Autodesk Inventor part; units mm, degrees
ref_plane "YZ Plane" through (0, 0, 0) normal (1, 0, 0) x (0, 1, 0)
ref_plane "XZ Plane" through (0, 0, 0) normal (0, 1, 0) x (-1, 0, 0)
ref_plane "XY Plane" through (0, 0, 0) normal (0, 0, 1) x (1, 0, 0)
sketch "Sketch1" plane through (0, 0, 0) normal (1, 0, 0) x (0, 1, 0)
  line L0 (-19.6181, -6.8872) -> (-0.5681, -6.8872)
  line L1 (-0.5681, -6.8872) -> (-0.5681, -10.0622)
  line L2 (-0.5681, -10.0622) -> (-19.6181, -10.0622)
  line L3 (-19.6181, -10.0622) -> (-19.6181, -6.8872)
  dimension "d7" = 19.05
  dimension "d8" = 3.175
extrude "Extrusion1" add sketch "Sketch1" along normal blind 38.1
sketch "Sketch2" plane through (0, -0.5681, -6.8872) normal (0, 1, 0) x (1, 0, 0)
  line L0 (38.1, 3.175) -> (38.1, 0)
  arc A0 (38.1, 1.5875) -> (241.3, 1.5875) centre (139.7, 115.1798) ccw
  line L1 (0, 0) -> (38.1, 0)
  point P0 (0, -6.8872)
  dimension "d11" = 203.2
  dimension "d12" = 152.4
  dimension "d17" = 1.5875
sketch "Sketch3" plane through (38.1, 0, 0) normal (1, 0, 0) x (0, 0, -1)
  line L0 (6.8872, -0.5681) -> (6.8872, -19.6181)
  line L1 (6.8872, -19.6181) -> (10.0622, -19.6181)
  line L2 (10.0622, -19.6181) -> (10.0622, -0.5681)
  line L3 (10.0622, -0.5681) -> (6.8872, -0.5681)
  point P0 (0, 0)
sweep "Sweep1" add profiles "Sketch3" path "Sketch2" path curves A0
sketch "Sketch4" plane through (0, -0.5681, -6.8872) normal (0, 1, 0) x (1, 0, 0)
  line L0 (239.7223, 1.7639) -> (242.8777, 1.4111)
  line L1 (0, 3.175) -> (38.1, 3.175)
  line L2 (239.7223, 1.7639) -> (239.7223, 20.8139)
  line L3 (239.7223, 20.8139) -> (242.8777, 20.8139)
  line L4 (242.8777, 20.8139) -> (242.8777, 1.4111)
  point P0 (0, -6.8872)
  dimension "d14" = 19.05
extrude "Extrusion2" add sketch "Sketch4" against normal blind 19.05
properties part number "RearSkidSteel"
The model under review builds one solid part; all positions refer to its coordinate system, in mm. A direction names the side the tool comes from. Give positions to 0.01 mm unless a question says otherwise; leave off trailing zeros. Order: outer loops, then holes, each group sorted by start corner. A loop starts at its lowest first (then second) coordinate and runs counter-clockwise, first axis right, second up. Notation, with made-up numbers: M 18,33.25 L 71,33.25 A26 cw 71,57.25 Z; hole C -19.75,81.25 d6. An arc over 180 degrees is marked long. One line per question, with ' | ' between items. Start each with the question number.
1) Consider section D-D, the plane z = 3. Give the boundary of the cut face in (x, y), then the cut area to 3 significant figures.
2) Clearance check with flat-ended pins moving along their axes: P1, Ø1.5, axis at y = -8.5, z = 20.5, coming from the -X side; P2, Ø9.5, axis at x = 18.5, y = -13.5, coming from the -Z side; P3, Ø2, axis at y = -13, z = 20, coming from the +X side; P4, Ø6, axis at y = -8.5, z = -7, coming from the +X side. State where each tip first meets the part, or that it passes through.
3) Consider section B-B, the plane z = 14. Give the boundary of the cut face in (x, y).
4) Wall thickness on L1, parallel to X at y = -5.25, z = -13; L2, parallel to Z at x = 12.5, y = -5.25; L3, parallel to X at y = -16.25, z = -3: over which ranges is each line inside the solid? List them lowest first. Write a range as from..to.
5) Consider section C-C, the plane z = -18. Give the boundary of the cut face in (x, y), then the cut area to 3 significant figures.
6) Mouldability with a two-part tool opening along X and no side actions: class faces 1 (the face through (19, -10, -6.887)), 2 (the face through (137.1, -9.96, 29.13)), 3 (the face through (142.327, -10.226, 31.497)) as pulls with the +X half, pulls with the -X half, needs draft (parallel to the pull), parting line crosses it, or undercut.
7) For faces 4 (the face through (242.878, -10, -18)), 5 (the face through (19, -10, -10.062)), list the 3-axis set-ups (+Z, -Z, +X, -X, +Y, -Y) from which the entire face can be reached by the end or side of a thin tool; tool diameter is ignored.
Found:
1) outline: M 50.55,-19.62 L 54.69,-19.62 L 54.69,-0.57 L 50.55,-0.57 Z; M 224.71,-19.62 L 228.85,-19.62 L 228.85,-0.57 L 224.71,-0.57 Z | area: 158 mm²
2) P1: stops at x = 80.73 | P2: stops at z = -10.06 | P3: stops at x = 200.44 | P4: stops at x = 242.88
3) outline: M 68.46,-19.62 L 73.72,-19.62 L 73.72,-0.57 L 68.46,-0.57 Z; M 205.68,-19.62 L 210.94,-19.62 L 210.94,-0.57 L 205.68,-0.57 Z
4) L1: x = 239.72..242.88 | L2: z = -10.06..-6.89 | L3: x = 42.68..46.48, 232.92..236.72
5) outline: M 239.72,-19.62 L 242.88,-19.62 L 242.88,-0.57 L 239.72,-0.57 Z | area: 60.1 mm²
6) face 1: needs draft | face 2: undercut | face 3: parting line crosses it
7) face 4: +Z, -Z, +X, +Y, -Y | face 5: -Z, -X, +Y, -Y
